from build123d import *

# Parameters (mm, degrees)
BOX020_W                = 12
BOX020_H                = 30
BOX020_DEPTH            = 8
BOX019_W                = 80
BOX019_H                = 3
BOX019_DEPTH            = 36
BODY007_PLACEMENT_ANGLE = 90


with BuildPart() as micro_usb_hole:
    # Box020 → Box020 (new body)
    with BuildSketch(Plane(origin=(0, -18.5, 4.7), x_dir=(0, -1, 0), z_dir=(0, 0, 1))):
        with Locations((6, 15)):
            Rectangle(BOX020_W, BOX020_H)
    extrude(amount=BOX020_DEPTH)


with BuildPart() as model_wall_with_micro_usb_clone:
    # Box019 → Box019 (new body)
    with BuildSketch(Plane(origin=(0, 0, 0), x_dir=(0, -1, 0), z_dir=(0, 0, 1))):
        with Locations((40, 1.5)):
            Rectangle(BOX019_W, BOX019_H)
    extrude(amount=BOX019_DEPTH)

    # Cut008: cut micro usb hole
    add(micro_usb_hole.part, mode=Mode.SUBTRACT)


with BuildPart() as model_wall_with_micro_usb_clone_1:
    # Cut008 placement: moved
    add(model_wall_with_micro_usb_clone.part.moved(Location((-12, 80, -3))))


with BuildPart() as model_wall_with_micro_usb_clone_2:
    # Body007 placement: moved
    add(model_wall_with_micro_usb_clone_1.part.rotate(Axis((0, 0, 0), (0, 1, 0)), BODY007_PLACEMENT_ANGLE))


solid = model_wall_with_micro_usb_clone_2.part
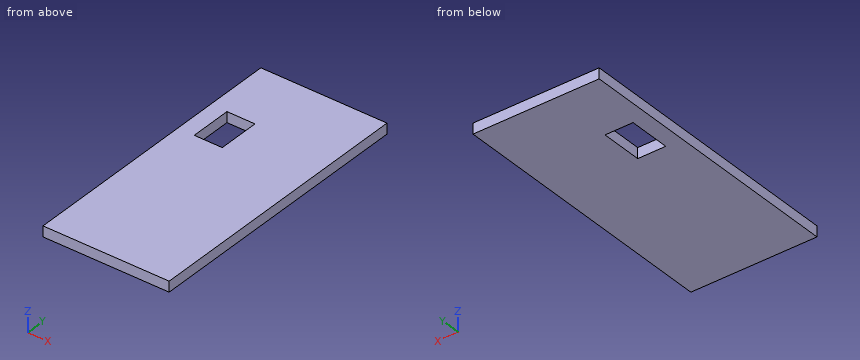
Geometry check sheet. Reference: the model listing, model coordinates, mm. Give positions to 0.01 mm unless a question says otherwise; leave off trailing zeros. Order: outer loops, then holes, each group sorted by start corner. A loop starts at its lowest first (then second) coordinate and runs counter-clockwise, first axis right, second up.
1) Cross-section at A-A (x = 7.5). Record the boundary of the cut face in (y, z), then the cut area to 3 significant figures.
Results are:
outline: (0, 9) - (49.5, 9) - (49.5, 12) - (0, 12) - close; (61.5, 9) - (80, 9) - (80, 12) - (61.5, 12) - close
area: 204 mm2
2) Material ranges on probe 1 along Y at (x, z) = (6, 11.75), recorded low to high.
Results are:
probe 1: y = 0 to 49.5, 61.5 to 80
3) Cross-section at B-B (y = 52). Record the boundary of the cut face in (x, z).
Results are:
outline: (-3, 9) - (1.7, 9) - (1.7, 12) - (-3, 12) - close; (9.7, 9) - (33, 9) - (33, 12) - (9.7, 12) - close
4) Cross-section at C-C (z = 9.8). Record the boundary of the cut face in (x, y), then the cut area to 3 significant figures.
Results are:
outline: (-3, 0) - (33, 0) - (33, 80) - (-3, 80) - close; hole (1.7, 49.5) - (9.7, 49.5) - (9.7, 61.5) - (1.7, 61.5) - close
area: 2,780 mm2
